Autodesk Inventor part; units mm, degrees
ref_plane "YZ Plane" through (0, 0, 0) normal (1, 0, 0) x (0, 1, 0)
ref_plane "XZ Plane" through (0, 0, 0) normal (0, 1, 0) x (-1, 0, 0)
ref_plane "XY Plane" through (0, 0, 0) normal (0, 0, 1) x (1, 0, 0)
sketch "Sketch1" plane through (0, 0, 0) normal (0, 0, 1) x (1, 0, 0)
  line L0 (0, 25.5) -> (5, 25.5)
  line L1 (5, 25.5) -> (5, -25.5)
  line L2 (5, -25.5) -> (0, -25.5)
  line L3 (0, -25.5) -> (0, 25.5)
  line L4 (5, 25.5) -> (7, 25.5)
  line L5 (7, 25.5) -> (7, -25.5)
  line L6 (7, -25.5) -> (5, -25.5)
  line L7 (5, -25.5) -> (5, 25.5)
  line L8 (7, 25.5) -> (9.8, 25.5)
  line L9 (9.8, 25.5) -> (9.8, -25.5)
  line L10 (9.8, -25.5) -> (7, -25.5)
  line L11 (7, -25.5) -> (7, 25.5)
  line L12 (9.8, -25.5) -> (11.8, -25.5)
  line L13 (11.8, -25.5) -> (11.8, 25.5)
  line L14 (11.8, 25.5) -> (9.8, 25.5)
  line L15 (9.8, 25.5) -> (9.8, -25.5)
  line L16 (0, 42.6516) -> (0, -39.217) construction
  line L17 (11.8, 25.5) -> (0, 25.5)
  line L18 (0, 25.5) -> (0, 27.5)
  line L19 (0, 27.5) -> (11.8, 27.5)
  line L20 (11.8, 27.5) -> (11.8, 25.5)
  line L21 (11.8, -25.5) -> (0, -25.5)
  line L22 (0, -25.5) -> (0, -27.5)
  line L23 (0, -27.5) -> (11.8, -27.5)
  line L24 (11.8, -27.5) -> (11.8, -25.5)
  point P0 (0, 0)
  point P1 (0, 0)
  dimension "d0" = 2
  dimension "d1" = 51
  dimension "d2" = 2.8
  dimension "d3" = 2
  dimension "d4" = 5
  dimension "d9" = 2
  dimension "d10" = 2
extrude "Extrusion1" add sketch "Sketch1" along normal blind 2 contours L0 L1 L2 L3 | L4 L5 L6 L1 | L8 L9 L10 L5 | L14 L13 L12 L9
extrude "Extrusion2" add sketch "Sketch1" along normal blind 8 contours L18 L19 L20 L14 L8 L4 L0 | L4 L5 L6 L1 | L2 L6 L10 L12 L24 L23 L22 | L14 L13 L12 L9
mirror "Mirror1" about plane through (0, 0, 0) normal (1, 0, 0) of "Extrusion1", "Extrusion2"
properties part number "BasicConnector"
Design review of the part built by this model. Coordinates are the model's own, in mm. A direction names the side the tool comes from. Give positions to 0.01 mm unless a question says otherwise; leave off trailing zeros. Write each loop counter-clockwise with the first axis right and the second up, starting at its lowest first coordinate (ties: lowest second). Pieces come first, ordered by that corner, then holes. Notation, with made-up numbers: (-20.75, 75) - (-0.75, 75) arc R32 ccw to (-0.75, 101) - close; hole circle Ø2 at (41, 10). An arc over 180 degrees is marked (long way). Return JSON: item names as keys, results as strings. Group by question number.
(1) We need section A-A, the plane z = 4.5. Give the boundary of the cut face in (x, y), then the cut area to 3 significant figures.
(2) Mouldability with a two-part tool opening along X and no side actions: class faces 3 (the flat face through (-11.8, 0, 4)), 4 (the flat face through (-5, 0, 5)), 5 (the flat face through (-5.4, 0.4, 8)) as +X half, -X half, draft (parallel to the pull), parting line (faces both ways), or undercut.
(3) Machinability: for faces 1 (the flat face through (-8, 25.5, 5)), 2 (the flat face through (0, -27.5, 4)), which of the approach directions +Z, -Z, +X, -X, +Y, -Y give a long, thin tool a straight path to every point of the face, cutting with its end or side? Answer none if there is none.
(4) We need section C-C, the plane y = -6.5. Give the boundary of the cut face in (x, z).
(5) To check wall thickness, follow probe 1 along X at (y, z) = (4, 7.5); probe 2 along Y at (x, z) = (-8.25, 4); probe 3 along Z at (x, y) = (4, 18). State the ranges of each line that lie inside material, in increasing order.
(6) We need section B-B, the plane x = 8.5. Give the boundary of the cut face in (y, z).
Reported:
{
 "1": {"outline": "(-11.8, -27.5) - (11.8, -27.5) - (11.8, 27.5) - (-11.8, 27.5) - close; hole (-9.8, -25.5) - (-7, -25.5) - (-7, 25.5) - (-9.8, 25.5) - close; hole (-5, -25.5) - (5, -25.5) - (5, 25.5) - (-5, 25.5) - close; hole (7, -25.5) - (9.8, -25.5) - (9.8, 25.5) - (7, 25.5) - close", "area": "502 mm2"},
 "2": {"face 3": "-X half", "face 4": "undercut", "face 5": "draft"},
 "3": {"face 1": "+Z", "face 2": "+Z, -Z, +X, -X, -Y"},
 "4": {"outline": "(-11.8, 0) - (11.8, 0) - (11.8, 8) - (9.8, 8) - (9.8, 2) - (7, 2) - (7, 8) - (5, 8) - (5, 2) - (-5, 2) - (-5, 8) - (-7, 8) - (-7, 2) - (-9.8, 2) - (-9.8, 8) - (-11.8, 8) - close"},
 "5": {"probe 1": "x = -11.8 to -9.8, -7 to -5, 5 to 7, 9.8 to 11.8", "probe 2": "y = -27.5 to -25.5, 25.5 to 27.5", "probe 3": "z = 0 to 2"},
 "6": {"outline": "(-27.5, 0) - (27.5, 0) - (27.5, 8) - (25.5, 8) - (25.5, 2) - (-25.5, 2) - (-25.5, 8) - (-27.5, 8) - close"}
}
